Build history of the part. All positions in model axes, mm. A direction names the side the tool comes from. Coordinates: 2 decimals unless noted, no trailing zeros. Order: outer loops, then holes, each group sorted by start corner. A loop starts at its lowest first (then second) coordinate and runs counter-clockwise, first axis right, second up. Notation, with made-up numbers: (79.5, -24.5) -> (91.5, -24.5) arc R4 cw to (91.5, -18.5) -> close; hole circle Ø11 at (67, -20.75). An arc over 180 degrees is marked (long way). Write each question's results on one line, items separated by ' | '.
from build123d import *

# Parameters (mm, degrees)
SKETCH1_W                      = 96
SKETCH1_H                      = 96
BOSS_EXTRUDE1_DEPTH            = 8
SKETCH2_W                      = 92
SKETCH2_H                      = 92
COMPONENT_PLATFORM_DEPTH       = 6
CABLE_SLOTS_DEPTH              = 6
SKETCH4_R                      = 7.5
CENTER_MASS_CUT_DEPTH          = 6
INNER_CORNER_FILLETS_R         = 3
SKETCH10_W                     = 11
SKETCH10_H                     = 10
MOTOR_CUTOUT_DEPTH             = 2
FILLET1_R                      = 3
M3X0_5_TAPPED_HOLE1_AT_2_COUNT = 2
M3X0_5_TAPPED_HOLE1_AT_2_PITCH = 70
M3X0_5_TAPPED_HOLE2_AT_2_COUNT = 2
M3X0_5_TAPPED_HOLE2_AT_2_PITCH = 70
M3X0_5_TAPPED_HOLE3_D          = 2.5
M3X0_5_TAPPED_HOLE3_DEPTH      = 7.5
M3X0_5_TAPPED_HOLE3_TIP        = 0.751075774
M2X0_4_TAPPED_HOLE1_D          = 1.6
M2X0_4_TAPPED_HOLE1_DEPTH      = 5.2
M2X0_4_TAPPED_HOLE1_TIP        = 0.480688495
M4X0_7_TAPPED_HOLE1_D          = 3.3


with BuildPart() as part:
    # Sketch1 → Boss-Extrude1 (new body)
    with BuildSketch(Plane.XY):
        Rectangle(SKETCH1_W, SKETCH1_H)
    extrude(amount=BOSS_EXTRUDE1_DEPTH)

    # Sketch2 → Component Platform (cut)
    with BuildSketch(Plane.XY.offset(8)):
        Rectangle(SKETCH2_W, SKETCH2_H)
    extrude(amount=-COMPONENT_PLATFORM_DEPTH, mode=Mode.SUBTRACT)

    # Sketch3 → Cable Slots (cut, symmetric)
    with BuildSketch(Plane.XY.offset(2)):
        with BuildLine():
            Line((-33.878679656, -25.121320344), (-28.878679656, -20.121320344))
            ThreePointArc((-28.878679656, -20.121320344), (-28.228361402, -19.148050297), (-28, -18))
            Line((-28, -18), (-28, 18))
            ThreePointArc((-28, 18), (-28.228361402, 19.148050297), (-28.878679656, 20.121320344))
            Line((-28.878679656, 20.121320344), (-33.878679656, 25.121320344))
            ThreePointArc((-33.878679656, 25.121320344), (-34.851949703, 25.771638598), (-36, 26))
            Line((-36, 26), (-48, 26))
            Line((-48, 26), (-48, -26))
            Line((-48, -26), (-36, -26))
            ThreePointArc((-36, -26), (-34.851949703, -25.771638598), (-33.878679656, -25.121320344))
        make_face()
        with BuildLine():
            Line((48, -26), (48, 26))
            Line((48, 26), (36, 26))
            ThreePointArc((36, 26), (34.851949703, 25.771638598), (33.878679656, 25.121320344))
            Line((33.878679656, 25.121320344), (28.878679656, 20.121320344))
            ThreePointArc((28.878679656, 20.121320344), (28.228361402, 19.148050297), (28, 18))
            Line((28, 18), (28, -18))
            ThreePointArc((28, -18), (28.228361402, -19.148050297), (28.878679656, -20.121320344))
            Line((28.878679656, -20.121320344), (33.878679656, -25.121320344))
            ThreePointArc((33.878679656, -25.121320344), (34.851949703, -25.771638598), (36, -26))
            Line((36, -26), (48, -26))
        make_face()
    extrude(amount=CABLE_SLOTS_DEPTH, both=True, mode=Mode.SUBTRACT)

    # Sketch4 → Center Mass Cut (cut)
    with BuildSketch(Plane.XY.offset(2)):
        Circle(SKETCH4_R)
    extrude(amount=-CENTER_MASS_CUT_DEPTH, mode=Mode.SUBTRACT)

    # Inner Corner Fillets
    inner_corner_fillets_edges = [part.edges().sort_by_distance(p)[0] for p in [
        (-46, -46, 5),
        (-46, 46, 5),
        (46, 46, 5),
        (46, -46, 5),
    ]]
    fillet(inner_corner_fillets_edges, radius=INNER_CORNER_FILLETS_R)

    # Sketch10 → Motor Cutout (cut)
    with BuildSketch(Plane.XY.offset(2)):
        with Locations((5.5, 0)):
            Rectangle(SKETCH10_W, SKETCH10_H)
    extrude(amount=-MOTOR_CUTOUT_DEPTH, mode=Mode.SUBTRACT)

    # Fillet1
    fillet1_edges = [part.edges().sort_by_distance(p)[0] for p in [
        (11, -5, 1),
        (11, 5, 1),
    ]]
    fillet(fillet1_edges, radius=FILLET1_R)

    # Sketch14 → M3x0.5 Tapped Hole1 (revolve, cut)
    with BuildSketch(Plane(origin=(48, -35, 5), x_dir=(0, 0, -1), z_dir=(0, 1, 0))):
        Polygon((0, 0), (0, 8.251075774), (1.25, 7.5), (1.25, 0), align=None)
    m3x0_5_tapped_hole1 = revolve(axis=Axis((54.35, -35, 5), (-1, 0, 0)), mode=Mode.SUBTRACT)

    # M3x0.5 Tapped Hole1 at 2: M3x0.5 Tapped Hole1 ×2
    with Locations(*[(0, i * M3X0_5_TAPPED_HOLE1_AT_2_PITCH, 0) for i in range(1, M3X0_5_TAPPED_HOLE1_AT_2_COUNT)]):
        add(m3x0_5_tapped_hole1, mode=Mode.SUBTRACT)

    # Sketch17 → M3x0.5 Tapped Hole2 (revolve, cut)
    with BuildSketch(Plane(origin=(35, 48, 5), x_dir=(0, 0, 1), z_dir=(1, 0, 0))):
        Polygon((0, 0), (0, 8.251075774), (1.25, 7.5), (1.25, 0), align=None)
    m3x0_5_tapped_hole2 = revolve(axis=Axis((35, 54.35, 5), (0, -1, 0)), mode=Mode.SUBTRACT)

    # M3x0.5 Tapped Hole2 at 2: M3x0.5 Tapped Hole2 ×2
    with Locations(*[(-i * M3X0_5_TAPPED_HOLE2_AT_2_PITCH, 0, 0) for i in range(1, M3X0_5_TAPPED_HOLE2_AT_2_COUNT)]):
        add(m3x0_5_tapped_hole2, mode=Mode.SUBTRACT)

    # Mirror1: M3x0.5 Tapped Hole1 across plane
    add(m3x0_5_tapped_hole1.mirror(Plane(origin=(0, 0, 0), x_dir=(0, 0, 1), z_dir=(1, 0, 0))), mode=Mode.SUBTRACT)

    # Mirror1 copy 1 sketch → Mirror1 copy 1 (revolve, cut)
    with BuildSketch(Plane(origin=(-48, 35, 5), x_dir=(0, 0, -1), z_dir=(0, 1, 0))):
        Polygon((0, 0), (0, -8.251075774), (1.25, -7.5), (1.25, 0), align=None)
    revolve(axis=Axis((-54.35, 35, 5), (-1, 0, 0)), mode=Mode.SUBTRACT)

    # Mirror2: M3x0.5 Tapped Hole2 across plane
    add(m3x0_5_tapped_hole2.mirror(Plane(origin=(0, 0, 0), x_dir=(0, 0, 1), z_dir=(0, -1, 0))), mode=Mode.SUBTRACT)

    # Mirror2 copy 1 sketch → Mirror2 copy 1 (revolve, cut)
    with BuildSketch(Plane(origin=(-35, -48, 5), x_dir=(0, 0, 1), z_dir=(1, 0, 0))):
        Polygon((0, 0), (0, -8.251075774), (1.25, -7.5), (1.25, 0), align=None)
    revolve(axis=Axis((-35, -54.35, 5), (0, -1, 0)), mode=Mode.SUBTRACT)

    # M3x0.5 Tapped Hole3
    with Locations(Plane.XY.offset(2)):
        with Locations((-26.5, -26.5), (26.5, -26.5), (26.5, 26.5), (-26.5, 26.5)):
            Hole(M3X0_5_TAPPED_HOLE3_D / 2, depth=M3X0_5_TAPPED_HOLE3_DEPTH)
            with Locations((0, 0, -(M3X0_5_TAPPED_HOLE3_DEPTH + M3X0_5_TAPPED_HOLE3_TIP / 2))):  # 118° drill point
                Cone(0, M3X0_5_TAPPED_HOLE3_D / 2, M3X0_5_TAPPED_HOLE3_TIP, mode=Mode.SUBTRACT)

    # M2x0.4 Tapped Hole1
    with Locations(Plane.XY.offset(2)):
        with Locations((6.72, -6.72), (0, -10), (-6.72, -6.72), (-10, 0), (-6.72, 6.72), (0, 10), (6.72, 6.72)):
            Hole(M2X0_4_TAPPED_HOLE1_D / 2, depth=M2X0_4_TAPPED_HOLE1_DEPTH)
            with Locations((0, 0, -(M2X0_4_TAPPED_HOLE1_DEPTH + M2X0_4_TAPPED_HOLE1_TIP / 2))):  # 118° drill point
                Cone(0, M2X0_4_TAPPED_HOLE1_D / 2, M2X0_4_TAPPED_HOLE1_TIP, mode=Mode.SUBTRACT)

    # M4x0.7 Tapped Hole1 (through all)
    with Locations(Plane.XY.offset(2)):
        with Locations((-3.74, -20.47), (11.5, -38.25)):
            Hole(M4X0_7_TAPPED_HOLE1_D / 2)


solid = part.part
Item 1: Slice it at B-B, the plane x = -15.5. List the corners of the cut face in (y, z), and give its area (3 significant figures).
Answer:
outline: (-48, 0) -> (48, 0) -> (48, 8) -> (46, 8) -> (46, 2) -> (-46, 2) -> (-46, 8) -> (-48, 8) -> close | area: 216 mm^2
Item 2: Drill centre lines: line 1 (Y direction, x = 26.5, z = 1.45); line 2 (X direction, y = 47.25, z = 5); line 3 (Y direction, x = -40, z = 4.75). Where is each one in solid material? Low to high. Write a range as from..to.
Answer:
line 1: y = -48..-27.75, -25.25..25.25, 27.75..48 | line 2: x = -48..-36.25, -33.75..33.75, 36.25..48 | line 3: y = -48..-46, 46..48
Item 3: Tool access for faces 1 (the flat face through (43.3, -26, 1.6)), 2 (the flat face through (-45, -26, 1)), 3 (the cylindrical face through (-47.01, -33.78, 5.27)), 4 (the flat face through (-11, 1, 2)): list every direction of +Z, -Z, +X, -X, +Y, -Y with a clear straight run to the whole face (end or side of a thin tool).
Answer:
face 1: +Z, -Z, +X | face 2: +Z, -Z, -X | face 3: +X, -X | face 4: +Z
Item 4: Slice it at A-A, the plane x = -39. List the corners of the cut face in (y, z).
Answer:
outline: (-48, 0) -> (-26, 0) -> (-26, 2) -> (-46, 2) -> (-46, 8) -> (-48, 8) -> close; (26, 0) -> (48, 0) -> (48, 8) -> (46, 8) -> (46, 2) -> (26, 2) -> close
Item 5: Pin check, flat tips, straight feed: pin 1 (5.5 mm diameter, centred on x = 11.5, y = -38.25, fed in from +Z); pin 2 (0.6 mm diameter, centred on y = 1, z = 1.5, fed in from -X). Stop position of each tip, or through.
Answer:
pin 1: stops at z = 2 | pin 2: stops at x = -28
Item 6: Slice it at C-C, the plane y = -13.5. List the corners of the cut face in (x, z).
Answer:
outline: (-28, 0) -> (28, 0) -> (28, 2) -> (-28, 2) -> close
Item 7: Pull direction X, two halves, no side cores. Call faces 5 (the cylindrical face through (-45.14, 45.1, 4.96)), 6 (the cylindrical face through (10.61, -36.86, 0.99)), 7 (the flat face through (48, -37, 4)), 8 (the flat face through (-48, -37, 4)): released by +X, released by -X, zero draft, split by the parting line, or undercut.
Answer:
face 5: undercut | face 6: undercut | face 7: released by +X | face 8: released by -X
